```python
from build123d import *

# Parameters (mm, degrees)
SKETCH_1_W          = 100
SKETCH_1_H          = 70
EXTRUDE_1_DEPTH     = 10
SKETCH_2_W          = 40
SKETCH_2_H          = 70
EXTRUDE_2_DEPTH     = 10
CUT_EXTRUDE_1_DEPTH = 81.777472107
SKETCH_4_W          = 50
SKETCH_4_H          = 40
EXTRUDE_3_DEPTH     = 5
EXTRUDE_START       = -5
SKETCH_5_W          = 50
SKETCH_5_H          = 40
EXTRUDE_4_DEPTH     = 5
SKETCH_6_R          = 5
EXTRUDE_5_DEPTH     = 30


with BuildPart() as part:
    # 草圖1 → 填料-伸長1 (new body)
    with BuildSketch(Plane.XY):
        Rectangle(SKETCH_1_W, SKETCH_1_H)
    extrude(amount=EXTRUDE_1_DEPTH)

    # 草圖2 → 填料-伸長2 (add)
    with BuildSketch(Plane.XY.offset(10)):
        Rectangle(SKETCH_2_W, SKETCH_2_H)
    extrude(amount=EXTRUDE_2_DEPTH)

    # 草圖3 → 除料-伸長1 (cut, through all)
    with BuildSketch(Plane(origin=(20, 0, 0), x_dir=(0, 0, -1), z_dir=(1, 0, 0))):
        with BuildLine():
            Line((-20, -35), (-20, -28))
            ThreePointArc((-20, -28), (-15.050252532, -30.050252532), (-13, -35))
            Line((-13, -35), (-20, -35))
        make_face()
    extrude(amount=-CUT_EXTRUDE_1_DEPTH, mode=Mode.SUBTRACT)

    # 草圖4 → 填料-伸長3 (add)
    with BuildSketch(Plane(origin=(20, 0, 0), x_dir=(0, 0, -1), z_dir=(1, 0, 0))):
        with Locations((-45, 15)):
            Rectangle(SKETCH_4_W, SKETCH_4_H)
        with BuildLine():
            Line((-70, 35), (-70, -5))
            ThreePointArc((-70, -5), (-90, 15), (-70, 35))
        make_face()
    extrude(amount=-EXTRUDE_3_DEPTH)

    # 草圖5 → 填料-伸長4 (add)
    with BuildSketch(Plane.ZY.offset(20).offset(EXTRUDE_START)):
        with Locations((45, 15)):
            Rectangle(SKETCH_5_W, SKETCH_5_H)
        with BuildLine():
            Line((70, 35), (70, -5))
            ThreePointArc((70, -5), (90, 15), (70, 35))
        make_face()
    extrude(amount=EXTRUDE_4_DEPTH)

    # 草圖6 → 填料-伸長5 (add)
    with BuildSketch(Plane(origin=(-15, 0, 0), x_dir=(0, 0, -1), z_dir=(1, 0, 0))):
        with Locations(Location((-70, 15, 0), (0, 0, 180))):
            Circle(SKETCH_6_R)
    extrude(amount=EXTRUDE_5_DEPTH)


solid = part.part
```
Verification items for the finished model (mm, model axes). A direction names the side the tool comes from. Give positions to 0.01 mm unless a question says otherwise; leave off trailing zeros. Loops run counter-clockwise (first coordinate to the right, second up) from the corner with the lowest first, then second, coordinate; pieces in that order, holes last. Notation, with made-up numbers: M 37,38.5 L 60,38.5 A28 ccw 60,56.5 Z; hole C 37,27 d4. An arc over 180 degrees is marked long. Return JSON: item names as keys, results as strings.
1) Material ranges on L1, parallel to X at y = 26.5, z = 37.5; L2, parallel to X at y = 8, z = 13; L3, parallel to Z at x = 30, y = -24, recorded low to high. Write a range as [from, to].
Findings:
{"L1": "x = [-20, -15], [15, 20]", "L2": "x = [-20, 20]", "L3": "z = [0, 10]"}
2) Mould release check, pull along X, two halves, no side actions. Record for faces 1 (the cylindrical face through (-0.21, 16.915, 74.619)), 2 (the flat face through (-50, 0, 5)), 3 (the flat face through (3.9, 35, 19.6)): released by +X, released by -X, zero draft, split by the parting line, or undercut.
Findings:
{"face 1": "undercut", "face 2": "released by -X", "face 3": "zero draft"}
3) Tool access check on faces 4 (the flat face through (18, -5, 45)), 5 (the flat face through (20, 16, 51)), 6 (the flat face through (50, 0, 5)), 7 (the flat face through (-1, 0, 0)), 8 (the flat face through (-20, 16, 41)). Record the directions out of +Z, -Z, +X, -X, +Y, -Y that give a thin tool (end or side, any length) a straight path to the whole face; none if there is none.
Findings:
{"face 4": "+Z, +X, -X, -Y", "face 5": "+Z, +X, +Y, -Y", "face 6": "+Z, -Z, +X, +Y, -Y", "face 7": "-Z, +X, -X, +Y, -Y", "face 8": "+Z, -X, +Y, -Y"}
4) Section check A-A, the plane z = 60. Enter the section's corners in (x, y).
Findings:
{"outline": "M -20,-5 L -15,-5 L -15,35 L -20,35 Z; M 15,-5 L 20,-5 L 20,35 L 15,35 Z"}
5) Section check B-B, the plane y = 15. Enter the section's corners in (x, z).
Findings:
{"outline": "M -50,0 L 50,0 L 50,10 L 20,10 L 20,90 L 15,90 L 15,75 L -15,75 L -15,90 L -20,90 L -20,10 L -50,10 Z; hole M -15,20 L 15,20 L 15,65 L -15,65 Z"}
6) Section check D-D, the plane y = 30.5. Enter the section's corners in (x, z).
Findings:
{"outline": "M -50,0 L 50,0 L 50,10 L 20,10 L 20,82.64 L 15,82.64 L 15,20 L -15,20 L -15,82.64 L -20,82.64 L -20,10 L -50,10 Z"}
7) Section check C-C, the plane x = -16.5. Enter the section's corners in (y, z).
Findings:
{"outline": "M -35,0 L 35,0 L 35,70 A20 ccw -5,70 L -5,20 L -28,20 A7 cw -35,13 Z"}
8) Gauge pin test, flat ends, axial feed: P1, Ø1.5, axis at x = 2, y = 9.5, coming from the -Z side; P2, Ø21, axis at y = 2, z = 59.5, coming from the -X side; P3, Ø1.5, axis at y = 1, z = 37.5, coming from the +X side; P4, Ø10, axis at x = -5.5, z = 24.5, coming from the -Y side. Record the tip position at first contact, or that the pin passes through.
Findings:
{"P1": "stops at z = 0", "P2": "stops at x = -20", "P3": "stops at x = 20", "P4": "stops at y = -28.02"}
